Autodesk Inventor part; units mm, degrees
ref_plane "YZ Plane" through (0, 0, 0) normal (1, 0, 0) x (0, 1, 0)
ref_plane "XZ Plane" through (0, 0, 0) normal (0, 1, 0) x (-1, 0, 0)
ref_plane "XY Plane" through (0, 0, 0) normal (0, 0, 1) x (1, 0, 0)
sketch "Sketch1" plane through (0, 0, 0) normal (0, 0, 1) x (1, 0, 0)
  line L0 (-50, -100) -> (50, -100)
  line L1 (50, -100) -> (50, 100)
  line L2 (50, 100) -> (-50, 100)
  line L3 (-50, 100) -> (-50, -100)
  line L4 (-50, -100) -> (50, 100) construction
  line L5 (50, -100) -> (-50, 100) construction
  line L6 (50, 100) -> (40, 100)
  line L7 (40, 100) -> (40, 90)
  line L8 (40, 90) -> (50, 90)
  line L9 (50, 90) -> (50, 100)
  line L10 (50, -100) -> (40, -100)
  line L11 (40, -100) -> (40, -90)
  line L12 (40, -90) -> (50, -90)
  line L13 (50, -90) -> (50, -100)
  point P0 (0, 0)
  dimension "d154" = 100
  dimension "d155" = 200
  dimension "d158" = 10
  dimension "d159" = 10
extrude "Plate5" add sketch "Sketch1" along normal blind 2 contours L3 L2 L7 L8 L1 L12 L11 L0
sketch "Sketch7" plane through (0, 0, 2) normal (0, 0, 1) x (1, 0, 0)
  circle A0 centre (-24.4419, 38.3162) radius 10
  point P0 (0, 0)
  dimension "d157" = 20
extrude "Cut1" cut sketch "Sketch7" against normal blind 2
sketch "Sketch8" plane through (0, 0, 2) normal (0, 0, 1) x (1, 0, 0)
  line L0 (-39.1312, 91.8227) -> (16.5981, 91.8227) construction
  line L1 (16.5981, 91.8227) -> (16.5981, 81.3689) construction
  line L2 (16.5981, 81.3689) -> (-39.1312, 81.3689) construction
  line L3 (-39.1312, 81.3689) -> (-39.1312, 91.8227) construction
  point P0 (0, 0)
mark "Mark2"
properties material "Stainless Steel"
Read the model definition and answer for the solid it produces. Units are mm, in the model's axes. Give positions to 0.01 mm unless a question says otherwise; leave off trailing zeros. Write each loop counter-clockwise with the first axis right and the second up, starting at its lowest first coordinate (ties: lowest second). Pieces come first, ordered by that corner, then holes. Notation, with made-up numbers: (-26.75, 38) -> (2.25, 38) arc R24 ccw to (2.25, 75) -> close; hole circle Ø5 at (71.25, -24). An arc over 180 degrees is marked (long way). Answer as a JSON object with one key per item and string values. Group by question number.
1) Find section B-B (x = -18.5). Write down the section's boundary in (y, z).
2) Find section A-A (y = 32). Write down the section's boundary in (x, z).
3) Each of these flat-tipped pins is pushed along its axis until it touches: P1, Ø1, axis at x = -20.5, y = -52, coming from the -Z side; P2, Ø16, axis at x = -24.44, y = 38.32, coming from the -Z side. Where does it stop, or does it pass through?
4) Find section C-C (z = 1.05). Write down the section's boundary in (x, y).
5) The mould has two halves that part along Y. Classify faces 1 (the flat face through (-1, 1, 0)), 2 (the cylindrical face through (-19.07, 46.75, 1.01)): +Y half, -Y half, draft (parallel to the pull), parting line (faces both ways), or undercut.
6) Consider L1, parallel to Y at x = 42, z = 1.9; L2, parallel to X at y = 36, z = 1.2. Determine where each line is inside the solid, lowest interval first. Write a range as from..to.
Values follow:
{
 "1": {"outline": "(-100, 0) -> (30.27, 0) -> (30.27, 2) -> (-100, 2) -> close; (46.36, 0) -> (100, 0) -> (100, 2) -> (46.36, 2) -> close"},
 "2": {"outline": "(-50, 0) -> (-32.19, 0) -> (-32.19, 2) -> (-50, 2) -> close; (-16.69, 0) -> (50, 0) -> (50, 2) -> (-16.69, 2) -> close"},
 "3": {"P1": "stops at z = 0", "P2": "passes through"},
 "4": {"outline": "(-50, -100) -> (40, -100) -> (40, -90) -> (50, -90) -> (50, 90) -> (40, 90) -> (40, 100) -> (-50, 100) -> close; hole circle Ø20 at (-24.44, 38.32)"},
 "5": {"face 1": "draft", "face 2": "undercut"},
 "6": {"L1": "y = -90..90", "L2": "x = -50..-34.17, -14.71..50"}
}
